Could you check a few things on this drawing? It's one solid part, dimensions in mm from its lowest x, y, z. A direction names the side the tool comes from. Round coordinates to 2 decimals unless told otherwise and drop trailing zeros. Write each loop counter-clockwise with the first axis right and the second up, starting at its lowest first coordinate (ties: lowest second). Pieces come first, ordered by that corner, then holes. Notation, with made-up numbers: (-20.5, -2.5) -> (30.5, -2.5) arc R18 cw to (30.5, 14.5) -> close; hole circle Ø6 at (-35.75, 73.5). An arc over 180 degrees is marked (long way). Answer in a Markdown table with one row per item.
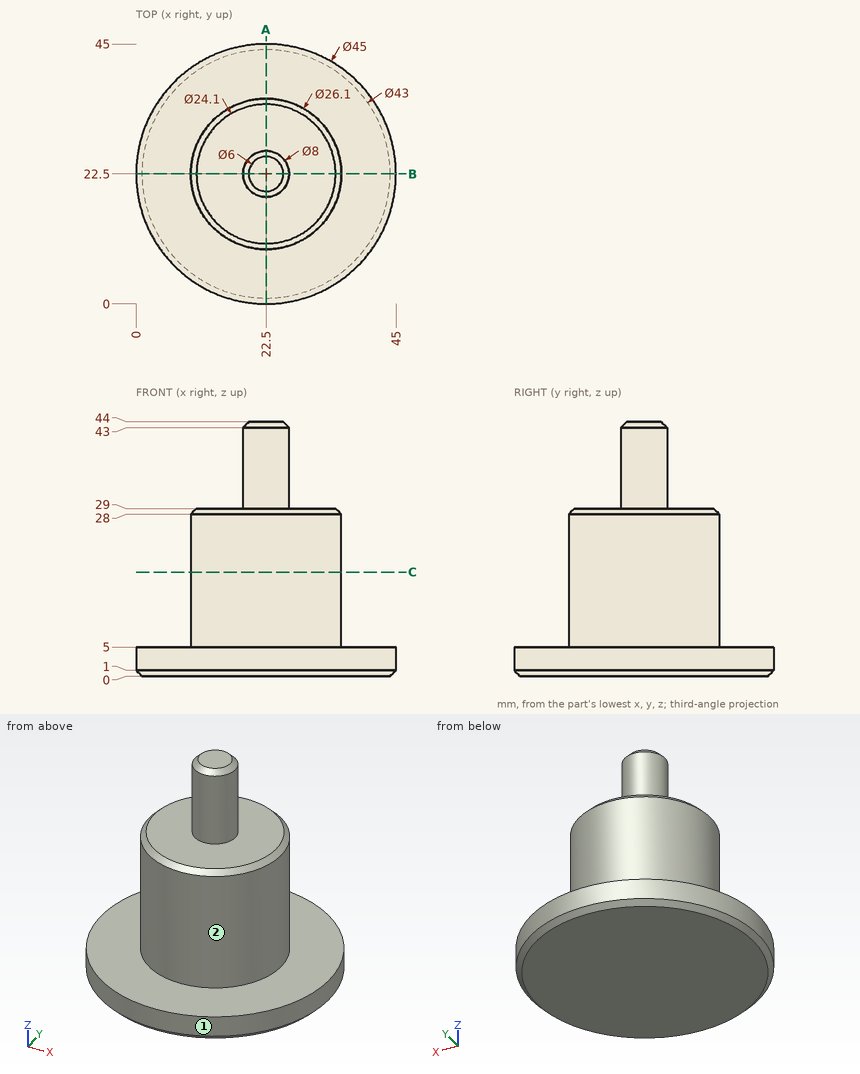
1) Please list where these lines run through material, in increasing order: line 1 (Y direction, x = 41.5, z = 2.5); line 2 (Z direction, x = 43, y = 21.5); line 3 (Z direction, x = 17, y = 12).
Findings:
| item | result |
|---|---|
| line 1 | y = 10.45 to 34.55 |
| line 2 | z = 0 to 5 |
| line 3 | z = 0 to 29 |
2) For pin 1 (2 mm diameter, centred on y = 21.5, z = 16, fed in from +X); pin 2 (3 mm diameter, centred on x = 24.5, z = 16, fed in from -Y); pin 3 (12 mm diameter, centred on x = 32.5, z = 27.5, fed in from -Y), each with a flat end and sliding along its axis, tell me the tip position at first contact or that it passes through.
Findings:
| item | result |
|---|---|
| pin 1 | stops at x = 35.55 |
| pin 2 | stops at y = 9.46 |
| pin 3 | stops at y = 10.08 |
3) Imagine slicing it at A-A, the plane x = 22.5. Please give me the cut outline in (y, z).
Findings:
| item | result |
|---|---|
| outline | (0, 1) -> (1, 0) -> (44, 0) -> (45, 1) -> (45, 5) -> (35.55, 5) -> (35.55, 28) -> (34.55, 29) -> (26.5, 29) -> (26.5, 43) -> (25.5, 44) -> (19.5, 44) -> (18.5, 43) -> (18.5, 29) -> (10.45, 29) -> (9.45, 28) -> (9.45, 5) -> (0, 5) -> close |
4) Imagine slicing it at C-C, the plane z = 18. Please give me the cut outline in (x, y), plus the area to 3 significant figures.
Findings:
| item | result |
|---|---|
| outline | circle Ø26.1 at (22.5, 22.5) |
| area | 535 mm^2 |
5) For the marked faces 1 and 2, which set-ups out of +Z, -Z, +X, -X, +Y, -Y let a thin tool reach every point of the face, with its end or its side?
Findings:
| item | result |
|---|---|
| face 1 | +Z, -Z |
| face 2 | +Z |
